from build123d import *

# Parameters (mm, degrees)
SKETCH1_W                    = 30
SKETCH1_H                    = 10.3
SKETCH1_W_2                  = 21
SKETCH1_H_2                  = 6.3
BOSS_EXTRUDE1_DEPTH          = 10.5
F_3_0_3_DIAMETER_HOLE1_D     = 3
SKETCH4_W                    = 30
SKETCH4_H                    = 10.3
SKETCH4_R                    = 2.425
BOSS_EXTRUDE2_DEPTH          = 2
CUT_EXTRUDE2_START           = -4
CUT_EXTRUDE2_DEPTH           = 4
CUT_EXTRUDE3_START           = -4
CUT_EXTRUDE3_DEPTH           = 4
MOVE_START                   = -10.6
MOVE_FACE1_OUTLINE_W         = 10.5
MOVE_FACE1_OUTLINE_H         = 6.5
MOVE_FACE1_DEPTH             = 21.2
MOVE_START_2                 = 7.55
MOVE_FACE1_2_OUTLINE_W       = 2
MOVE_FACE1_2_OUTLINE_H       = 4.2
MOVE_FACE1_2_DEPTH           = 2.162306716
BOSS_EXTRUDE3_START          = 1.5
BOSS_EXTRUDE3_DEPTH          = 1.5
CUT_EXTRUDE4_DEPTH           = 2
DELETEFACE1_START            = 10.5
DELETEFACE1_DEPTH            = 2
CHAMFER1_SIZE                = 0.5
SKETCH10_R                   = 3.5
CUT_EXTRUDE5_DEPTH           = 10.3
CUT_EXTRUDE5_DRAFT           = -3
CUT_EXTRUDE5_PROFILE_2_DEPTH = 10.3
CUT_EXTRUDE5_PROFILE_2_DRAFT = -3


# Read off the part's stored shape, not the designer's step: Move Face1, DeleteFace1
with BuildPart() as part:
    # Sketch1 → Boss-Extrude1 (new body)
    with BuildSketch(Plane(origin=(0, 0, 0), x_dir=(1, 0, 0), z_dir=(0, 1, 0))):
        Rectangle(SKETCH1_W, SKETCH1_H)
        Rectangle(SKETCH1_W_2, SKETCH1_H_2, mode=Mode.SUBTRACT)
    extrude(amount=BOSS_EXTRUDE1_DEPTH)

    # Ø3.0 (3) Diameter Hole1 (through all)
    with Locations(Plane.XY.offset(5.15)):
        with Locations((-4.699, 6), (4.699, 6)):
            Hole(F_3_0_3_DIAMETER_HOLE1_D / 2)

    # Sketch4 → Boss-Extrude2 (add)
    with BuildSketch(Plane(origin=(0, 10.5, 0), x_dir=(1, 0, 0), z_dir=(0, 1, 0))):
        Rectangle(SKETCH4_W, SKETCH4_H)
        with Locations(Location((-10.925, 0, 0), (0, 0, 79.906343141))):
            Circle(SKETCH4_R, mode=Mode.SUBTRACT)
        with Locations(Location((10.925, 0, 0), (0, 0, 100.093656859))):
            Circle(SKETCH4_R, mode=Mode.SUBTRACT)
        with Locations(Location((3.425, 0, 0), (0, 0, 270))):
            Circle(SKETCH4_R, mode=Mode.SUBTRACT)
    extrude(amount=BOSS_EXTRUDE2_DEPTH)

    # Sketch5 → Cut-Extrude2 (cut)
    with BuildSketch(Plane(origin=(0, 12.5, 0), x_dir=(1, 0, 0), z_dir=(0, 1, 0)).offset(CUT_EXTRUDE2_START)):
        with BuildLine():
            Line((-7.65, 2), (-8.4, 2))
            Line((-8.4, 2), (-9.553641185, 2))
            ThreePointArc((-9.553641185, 2), (-8.779519852, 1.130283122), (-8.5, 0))
            ThreePointArc((-8.5, 0), (-8.779519852, -1.130283122), (-9.553641185, -2))
            Line((-9.553641185, -2), (-8.4, -2))
            Line((-8.4, -2), (-7.65, -2))
            Line((-7.65, -2), (-7.65, 2))
        make_face()
    cut_extrude2 = extrude(amount=CUT_EXTRUDE2_DEPTH, mode=Mode.SUBTRACT)

    # Sketch6 → Cut-Extrude3 (cut)
    with BuildSketch(Plane(origin=(0, 12.5, 0), x_dir=(1, 0, 0), z_dir=(0, 1, 0)).offset(CUT_EXTRUDE3_START)):
        with BuildLine():
            Line((2.053641185, 2), (1, 2))
            Line((1, 2), (0.4, 2))
            Line((0.4, 2), (0.4, -2))
            Line((0.4, -2), (1, -2))
            Line((1, -2), (2.053641185, -2))
            ThreePointArc((2.053641185, -2), (1, 0), (2.053641185, 2))
        make_face()
    extrude(amount=CUT_EXTRUDE3_DEPTH, mode=Mode.SUBTRACT)

    # Mirror1: Cut-Extrude2 across plane
    add(cut_extrude2.mirror(Plane(origin=(0, 0, 0), x_dir=(0, 0, 1), z_dir=(1, 0, 0))), mode=Mode.SUBTRACT)

    # Move Face1 outline → Move Face1 (cut)
    with BuildSketch(Plane.YZ.offset(MOVE_START)):
        with Locations((5.25, 0)):
            Rectangle(MOVE_FACE1_OUTLINE_W, MOVE_FACE1_OUTLINE_H)
    extrude(amount=MOVE_FACE1_DEPTH, mode=Mode.SUBTRACT)

    # Move Face1 2 outline → Move Face1 2 (cut)
    with BuildSketch(Plane.YZ.offset(MOVE_START_2)):
        with Locations((11.5, 0)):
            Rectangle(MOVE_FACE1_2_OUTLINE_W, MOVE_FACE1_2_OUTLINE_H)
    extrude(amount=MOVE_FACE1_2_DEPTH, mode=Mode.SUBTRACT)

    # Sketch7 → Boss-Extrude3 (add)
    # profile 1 of 4: a face of its own
    with BuildSketch(Plane.XZ.offset(-10.5).offset(BOSS_EXTRUDE3_START)):
        with BuildLine():
            Line((9.712306716, -2.1), (7.55, -2.1))
            Line((7.55, -2.1), (7.55, 2.1))
            Line((7.55, 2.1), (9.712306716, 2.1))
            ThreePointArc((9.712306716, 2.1), (10.141357197, 2.294891927), (10.6, 2.403122968))
            Line((10.6, 2.403122968), (10.6, 3.25))
            Line((10.6, 3.25), (-10.6, 3.25))
            Line((-10.6, 3.25), (-10.6, 2.403122968))
            ThreePointArc((-10.6, 2.403122968), (-10.053199943, 2.262871994), (-9.553641185, 2))
            Line((-9.553641185, 2), (-7.65, 2))
            Line((-7.65, 2), (-7.65, -2))
            Line((-7.65, -2), (-9.553641185, -2))
            ThreePointArc((-9.553641185, -2), (-10.053199943, -2.262871994), (-10.6, -2.403122968))
            Line((-10.6, -2.403122968), (-10.6, -3.25))
            Line((-10.6, -3.25), (10.6, -3.25))
            Line((10.6, -3.25), (10.6, -2.403122968))
            ThreePointArc((10.6, -2.403122968), (10.141357197, -2.294891927), (9.712306716, -2.1))
        make_face()
        with BuildLine():
            Line((0.4, -2), (0.4, 2))
            Line((0.4, 2), (2.053641185, 2))
            ThreePointArc((2.053641185, 2), (5.85, 0), (2.053641185, -2))
            Line((2.053641185, -2), (0.4, -2))
        make_face(mode=Mode.SUBTRACT)
    # profile 2 of 4: a face of its own
    with BuildSketch(Plane.XZ.offset(-10.5).offset(BOSS_EXTRUDE3_START)):
        with BuildLine():
            Line((2.053641185, 2), (2.053641185, -2))
            ThreePointArc((2.053641185, -2), (5.85, 0), (2.053641185, 2))
        make_face()
    # profile 3 of 4: a face of its own
    with BuildSketch(Plane.XZ.offset(-10.5).offset(BOSS_EXTRUDE3_START)):
        with BuildLine():
            Line((-9.553641185, 2), (-9.553641185, -2))
            ThreePointArc((-9.553641185, -2), (-10.053199943, -2.262871994), (-10.6, -2.403122968))
            Line((-10.6, -2.403122968), (-10.6, 2.403122968))
            ThreePointArc((-10.6, 2.403122968), (-10.053199943, 2.262871994), (-9.553641185, 2))
        make_face()
    # profile 4 of 4: a face of its own
    with BuildSketch(Plane.XZ.offset(-10.5).offset(BOSS_EXTRUDE3_START)):
        with BuildLine():
            Line((10.6, 2.403122968), (10.6, -2.403122968))
            ThreePointArc((10.6, -2.403122968), (10.141357197, -2.294891927), (9.712306716, -2.1))
            Line((9.712306716, -2.1), (9.712306716, 2.1))
            ThreePointArc((9.712306716, 2.1), (10.141357197, 2.294891927), (10.6, 2.403122968))
        make_face()
    extrude(amount=-BOSS_EXTRUDE3_DEPTH)

    # Sketch9 → Cut-Extrude4 (cut)
    with BuildSketch(Plane(origin=(0, 12.5, 0), x_dir=(1, 0, 0), z_dir=(0, 1, 0))):
        Polygon((-12.325074403, 2.425), (-13.725148806, 0), (-12.325074403, -2.425), (-9.524925597, -2.425), (-8.124851194, 0), (-9.524925597, 2.425), align=None)
        Polygon((1, 1.400074403), (1, -1.400074403), (3.425, -2.800148806), (5.85, -1.400074403), (5.85, 1.400074403), (3.425, 2.800148806), align=None)
        Polygon((11.64973184, 2.704736049), (8.944995791, 1.980004209), (8.220263951, -0.72473184), (10.20026816, -2.704736049), (12.905004209, -1.980004209), (13.629736049, 0.72473184), align=None)
    extrude(amount=-CUT_EXTRUDE4_DEPTH, mode=Mode.SUBTRACT)

    # DeleteFace1 outline → DeleteFace1 (add)
    with BuildSketch(Plane(origin=(0, 0, 0), x_dir=(1, 0, 0), z_dir=(0, 1, 0)).offset(DELETEFACE1_START)):
        Polygon((9.392826181, 2.1), (9.712306716, 2.1), (9.712306716, -2.1), (9.595532111, -2.1), (10.20026816, -2.704736049), (12.905004209, -1.980004209), (13.629736049, 0.72473184), (11.64973184, 2.704736049), align=None)
    extrude(amount=DELETEFACE1_DEPTH)

    # Chamfer1
    chamfer1_edges = [part.edges().sort_by_distance(p)[0] for p in [
        (8.631153358, 12.5, 2.1),
        (7.55, 12.5, 0),
        (8.631153358, 12.5, -2.1),
        (1.219550808, 12.5, 2),
        (-8.464775866, 12.5, -2),
        (-10.925, 12.5, 2.425),
        (-9.402238665, 12.5, 2.2125),
        (-13.025111604, 12.5, 1.2125),
        (-13.025111604, 12.5, -1.2125),
        (-10.925, 12.5, -2.425),
        (-9.402238665, 12.5, -2.2125),
        (2.732050808, 12.5, 2.400074403),
        (4.6375, 12.5, 2.100111604),
        (5.85, 12.5, 0),
        (4.6375, 12.5, -2.100111604),
        (2.732050808, 12.5, -2.400074403),
        (9.712306716, 12.5, 0),
        (0, 12.5, -5.15),
        (-15, 12.5, 0),
        (0, 12.5, 5.15),
        (15, 12.5, 0),
        (-7.65, 12.5, 0),
        (-8.464775866, 12.5, 2),
        (0.4, 12.5, 0),
        (1.219550808, 12.5, -2),
    ]]
    chamfer(chamfer1_edges, length=CHAMFER1_SIZE)


with BuildPart() as cut_extrude5_tool:
    # Sketch10 → Cut-Extrude5 (with draft: the straight prism first)
    with BuildSketch(Plane(origin=(0, 0, -5.15), x_dir=(-1, 0, 0), z_dir=(0, 0, -1))):
        with Locations((16, 5.45673788)):
            Circle(SKETCH10_R)
    extrude(amount=-CUT_EXTRUDE5_DEPTH)
    # Cut-Extrude5: the draft: its side faces are tilted about the plane it starts from
    cut_extrude5_sides = [cut_extrude5_tool.faces().sort_by_distance(p)[0] for p in [
        (-12.5, 5.45673788, 0),
    ]]
    draft(cut_extrude5_sides, Plane(origin=(0, 0, -5.15), x_dir=(-1, 0, 0), z_dir=(0, 0, -1)), CUT_EXTRUDE5_DRAFT)


with BuildPart() as part_1:
    add(part.part)

    # Cut-Extrude5: cut by cut_extrude5_tool
    add(cut_extrude5_tool.part, mode=Mode.SUBTRACT)


with BuildPart() as cut_extrude5_profile_2_tool:
    # Sketch10 → Cut-Extrude5 profile 2 (with draft: the straight prism first)
    with BuildSketch(Plane(origin=(0, 0, -5.15), x_dir=(-1, 0, 0), z_dir=(0, 0, -1))):
        with Locations((-16, 5.45673788)):
            Circle(SKETCH10_R)
    extrude(amount=-CUT_EXTRUDE5_PROFILE_2_DEPTH)
    # Cut-Extrude5 profile 2: the draft: its side faces are tilted about the plane it starts from
    cut_extrude5_profile_2_sides = [cut_extrude5_profile_2_tool.faces().sort_by_distance(p)[0] for p in [
        (19.5, 5.45673788, 0),
    ]]
    draft(cut_extrude5_profile_2_sides, Plane(origin=(0, 0, -5.15), x_dir=(-1, 0, 0), z_dir=(0, 0, -1)), CUT_EXTRUDE5_PROFILE_2_DRAFT)


with BuildPart() as part_2:
    add(part_1.part)

    # Cut-Extrude5 profile 2: cut by cut_extrude5_profile_2_tool
    add(cut_extrude5_profile_2_tool.part, mode=Mode.SUBTRACT)


solid = part_2.part
Source: CAD feature listing. Evaluate the final solid. Frame: model axes, mm. A direction names the side the tool comes from. Coordinates: 2 decimals unless noted, no trailing zeros. Loops run counter-clockwise (first coordinate to the right, second up) from the corner with the lowest first, then second, coordinate; pieces in that order, holes last. Notation, with made-up numbers: (2.5, 81) -> (30.5, 81) arc R16 cw to (30.5, 97) -> close; hole circle Ø8 at (-40, 43). An arc over 180 degrees is marked (long way). Answer in a Markdown table with one row per item. Add a question column.
Q1. Section B-B on x = -4. Return the cut outline in (y, z), and give its area (3 significant figures).
Q2. Reachability of faces 5 (the face through (7.55, 10, 0)), 6 (the face through (-15, 10, 0)), 7 (the face through (-13.25, 12.25, -1.32)) from +Z, -Z, +X, -X, +Y, -Y: full face, straight path, thin tool, end or side. Return the list, or none.
Q3. Ray query, line 1 along Z through (x, y) = (5, 8); line 2 along Y through (x, z) = (-6.5, 2.5). Return the intervals inside material, ascending.
Q4. Section C-C on y = 6.5. Give the number of separate pieces and of enclosed holes in the cut face, and give its area (3 significant figures).
Q5. Pull-direction query (X, two-part tool) for faces 1 (the face through (15, 1, 0)), 2 (the face through (-13.23, 12.25, 1.36)), 3 (the face through (0, 12.5, -3)), 4 (the face through (-3.2, 6.07, 4.19)); classes: pulls with the +X half, pulls with the -X half, needs draft (parallel to the pull), parting line crosses it, or undercut.
Q6. Section A-A on z = -4. Return the cut outline in (x, y).
Q7. Contact query for flat-ended pins moving along their axis: pin 1 Ø1.1 at (x, z) = (3, 1) entering from +Y; pin 2 Ø1.5 at (x, z) = (-8, 0) entering from -Y. Output: stop coordinate, or through.
Computed values:
| question | item | result |
|---|---|---|
| 1 | outline | (0, -5.15) -> (4.67, -5.15) -> (4.67, -3.25) -> (0, -3.25) -> close; (0, 3.25) -> (4.67, 3.25) -> (4.67, 5.15) -> (0, 5.15) -> close; (7.33, -5.15) -> (12, -5.15) -> (12.5, -4.65) -> (12.5, 4.65) -> (12, 5.15) -> (7.33, 5.15) -> (7.33, 3.25) -> (9, 3.25) -> (9, -3.25) -> (7.33, -3.25) -> close |
| 1 | area | 59.9 mm^2 |
| 2 | face 5 | +Y, -Y |
| 2 | face 6 | +Z, -Z, -X, +Y, -Y |
| 2 | face 7 | +Y |
| 3 | line 1 | z = -5.15 to -3.25, 3.25 to 5.15 |
| 3 | line 2 | y = 9 to 12.5 |
| 4 | separate pieces | 4 |
| 4 | enclosed holes | 0 |
| 4 | area | 107 mm^2 |
| 5 | face 1 | pulls with the +X half |
| 5 | face 2 | undercut |
| 5 | face 3 | needs draft |
| 5 | face 4 | undercut |
| 6 | outline | (-15, 0) -> (15, 0) -> (15, 2.17) arc R3.44 cw to (15, 8.75) -> (15, 12) -> (14.5, 12.5) -> (-14.5, 12.5) -> (-15, 12) -> (-15, 8.75) arc R3.44 cw to (-15, 2.17) -> close; hole circle Ø3 at (-4.7, 6); hole circle Ø3 at (4.7, 6) |
| 7 | pin 1 | stops at y = 10.5 |
| 7 | pin 2 | stops at y = 9 |
